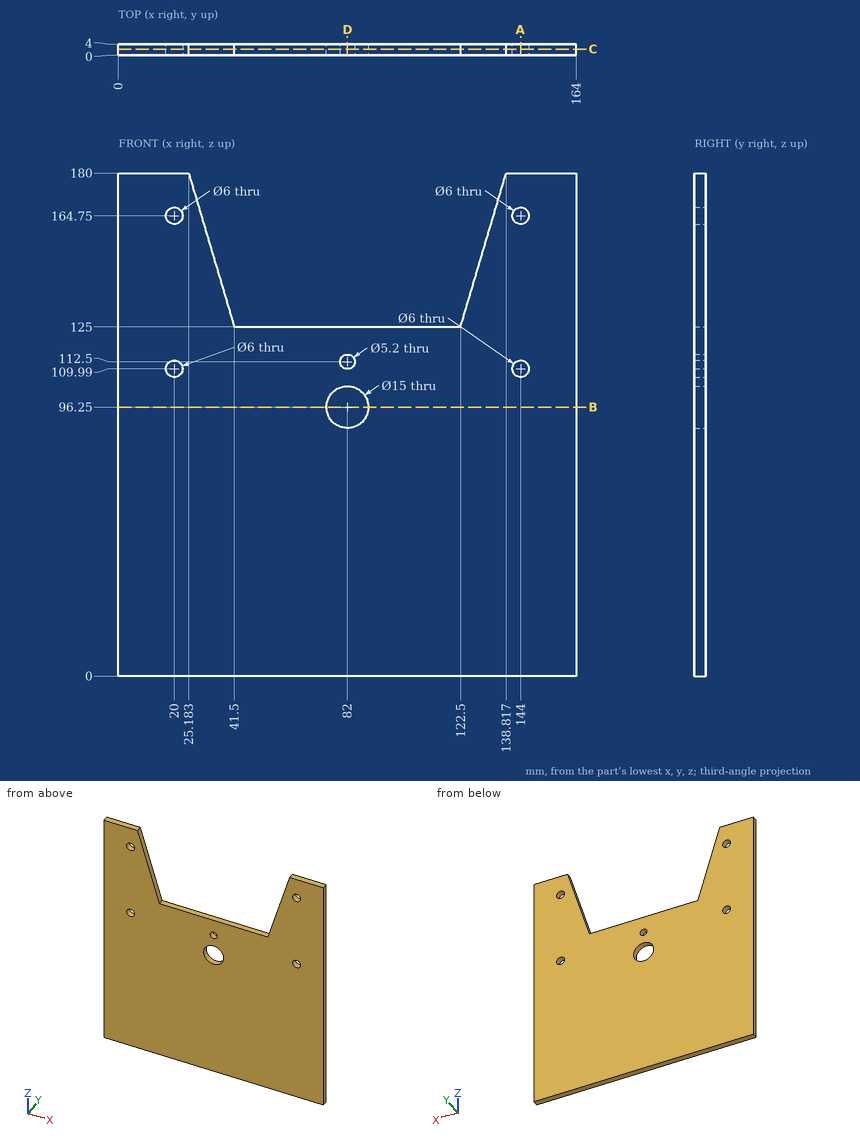
Answer from the drawing. Dimensions are ordinates in mm from the lowest x, y and z of the part. Give positions to 0.01 mm unless a question says otherwise; leave off trailing zeros. Order: outer loops, then holes, each group sorted by start corner. A loop starts at its lowest first (then second) coordinate and runs counter-clockwise, first axis right, second up. Notation, with made-up numbers: (46.25, 75.25) - (102.25, 75.25) arc R18 ccw to (102.25, 105.25) - close; hole circle Ø7 at (-9.5, 38.25). An arc over 180 degrees is marked (long way). Use one line per item in the form item = value.
1) Each of these flat-tipped pins is pushed along its axis until it touches: pin 1 (5 mm diameter, centred on x = 20, z = 109.99, fed in from -Y); pin 2 (1.2 mm diameter, centred on x = 70.5, y = 1.5, fed in from +Z). Where does it stop, or does it pass through?
Verdict:
pin_1 = through
pin_2 = 125
2) Consider probe 1 along Z at (x, y) = (82, 2.5); probe 2 along Z at (x, y) = (20, 1.8); probe 3 along X at (y, z) = (2.85, 96.25). Determine where each line is inside the solid, lowest interval first. Write a range as [from, to].
Verdict:
probe_1 = [0, 88.75], [103.75, 109.9], [115.1, 125]
probe_2 = [0, 106.99], [112.99, 161.75], [167.75, 180]
probe_3 = [0, 74.5], [89.5, 164]
3) Find section C-C on y = 2.2. Determine the outline of the cut face in (x, z).
Verdict:
outline = (0, 0) - (164, 0) - (164, 180) - (138.82, 180) - (122.5, 125) - (41.5, 125) - (25.18, 180) - (0, 180) - close; hole circle Ø6 at (20, 109.99); hole circle Ø6 at (20, 164.75); hole circle Ø15 at (82, 96.25); hole circle Ø5.2 at (82, 112.5); hole circle Ø6 at (144, 109.99); hole circle Ø6 at (144, 164.75)
4) Find section A-A on x = 144. Determine the outline of the cut face in (y, z).
Verdict:
outline = (0, 0) - (4, 0) - (4, 106.99) - (0, 106.99) - close; (0, 112.99) - (4, 112.99) - (4, 161.75) - (0, 161.75) - close; (0, 167.75) - (4, 167.75) - (4, 180) - (0, 180) - close
5) Find section D-D on x = 82. Determine the outline of the cut face in (y, z).
Verdict:
outline = (0, 0) - (4, 0) - (4, 88.75) - (0, 88.75) - close; (0, 103.75) - (4, 103.75) - (4, 109.9) - (0, 109.9) - close; (0, 115.1) - (4, 115.1) - (4, 125) - (0, 125) - close
6) Find section B-B on z = 96.25. Determine the outline of the cut face in (x, y).
Verdict:
outline = (0, 0) - (74.5, 0) - (74.5, 4) - (0, 4) - close; (89.5, 0) - (164, 0) - (164, 4) - (89.5, 4) - close
